Could you check a few things on this model? Use its own coordinates, in mm. Face numbers are marked on the shaded views. A direction names the side the tool comes from. Round coordinates to 2 decimals unless told otherwise and drop trailing zeros. Loops run counter-clockwise (first coordinate to the right, second up) from the corner with the lowest first, then second, coordinate; pieces in that order, holes last. Notation, with made-up numbers: (39.25, 16) -> (94.25, 16) arc R21 ccw to (94.25, 24) -> close; hole circle Ø3 at (54, 73.5). An arc over 180 degrees is marked (long way). Write each question's results on one line, items separated by ' | '.
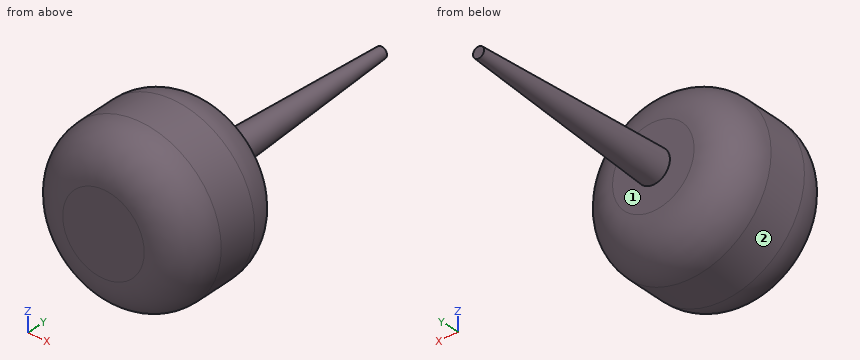
from build123d import *

# Parameters (mm, degrees)
F0_R     = 10
F1_DEPTH = 15
F2_R     = 5.08
F3_R     = 2
F4_DEPTH = 25.4
F4_TAPER = 3


with BuildPart() as f1:
    # F0 (on Front) → F1 (new body)
    with BuildSketch(Plane.XZ):
        Circle(F0_R)
    extrude(amount=-F1_DEPTH)

    # F2
    f2_edges = [f1.edges().sort_by_distance(p)[0] for p in [
        (-10, 0, 0),
        (-10, 15, 0),
    ]]
    fillet(f2_edges, radius=F2_R)

    # F3 (on face) → F4 (join)
    with BuildSketch(Plane(origin=(0, 15, 0), x_dir=(-1, 0, 0), z_dir=(0, 1, 0))):
        Circle(F3_R)
    extrude(amount=F4_DEPTH, taper=F4_TAPER)


solid = f1.part
1) I want a section at B-B, the plane y = 26.5. Write out the boundary of the cut face in (x, z), plus the area to 3 significant figures.
Model answer:
outline: circle Ø2.79 at (0, 0) | area: 6.13 mm2
2) I need wall thicknesses on line 1 (Y direction, x = 2.5, z = 3.5); line 2 (Z direction, x = -3, y = 14.5); line 3 (Z direction, x = 6.5, y = 2.5). Which ranges of each line are inside material? Lowest first, please.
Model answer:
line 1: y = 0 to 15 | line 2: z = -6.45 to 6.45 | line 3: z = -6.65 to 6.65
3) I want a section at A-A, the plane y = 8. Write out the boundary of the cut face in (x, z), plus the area to 3 significant figures.
Model answer:
outline: circle Ø20 at (0, 0) | area: 314 mm2
4) For the marked faces 1 and 2, which set-ups out of +Z, -Z, +X, -X, +Y, -Y let a thin tool reach every point of the face, with its end or its side?
Model answer:
face 1: +Y | face 2: +Y, -Y
5) I'm going to push flat-ended pins straight in: pin 1 (4 mm diameter, centred on x = 7, y = 7.5, fed in from +Z); pin 2 (12 mm diameter, centred on x = 1, z = -5, fed in from +Y); pin 3 (1.5 mm diameter, centred on y = 34, z = -0.5, fed in from -X); pin 4 (2 mm diameter, centred on x = 3.5, z = -2.5, fed in from +Y). Where does each tip first touch, or does it pass through?
Model answer:
pin 1: stops at z = 8.66 | pin 2: stops at y = 40.4 | pin 3: stops at x = -1.03 | pin 4: stops at y = 15
